The model under review builds one solid part; all positions refer to its coordinate system, in mm. Face numbers are marked on the shaded views. A direction names the side the tool comes from. Round coordinates to 2 decimals unless told otherwise and drop trailing zeros. Loops run counter-clockwise (first coordinate to the right, second up) from the corner with the lowest first, then second, coordinate; pieces in that order, holes last. Notation, with made-up numbers: M 1.25,73.5 L 57.25,73.5 A21 ccw 57.25,88.5 Z; hole C 25.5,-17.75 d3. An arc over 180 degrees is marked long. One line per question, with ' | ' between items.
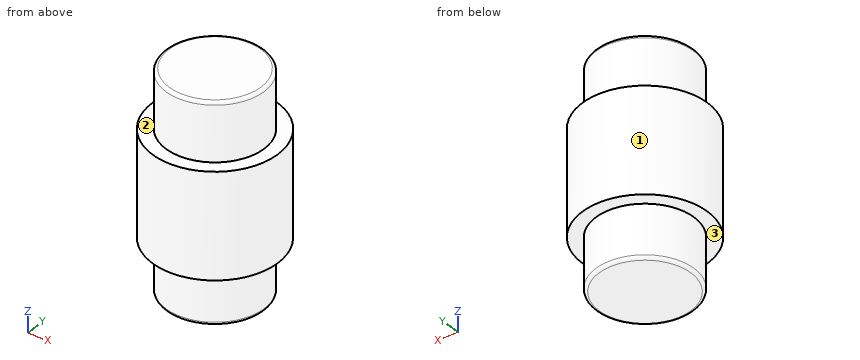
Autodesk Inventor part; units mm, degrees
ref_plane "YZ Plane" through (0, 0, 0) normal (1, 0, 0) x (0, 1, 0)
ref_plane "XZ Plane" through (0, 0, 0) normal (0, 1, 0) x (-1, 0, 0)
ref_plane "XY Plane" through (0, 0, 0) normal (0, 0, 1) x (1, 0, 0)
sketch "Sketch1" plane through (0, 0, 0) normal (0, 0, 1) x (1, 0, 0)
  circle A0 centre (0, 0) radius 4.7
  dimension "d0" = 9.4
extrude "Extrusion1" add sketch "Sketch1" along normal blind 5
sketch "Sketch2" plane through (0, 0, 5) normal (0, 0, 1) x (1, 0, 0)
  circle A0 centre (0, 0) radius 6
  dimension "d3" = 12
extrude "Extrusion2" add sketch "Sketch2" along normal blind 10
sketch "Sketch3" plane through (0, 0, 15) normal (0, 0, 1) x (1, 0, 0)
  circle A0 centre (0, 0) radius 4.7
  dimension "d6" = 9.4
extrude "Extrusion3" add sketch "Sketch3" along normal blind 5.556
fillet "Fillet1" radius 0.3 2 edges at (-4.7, 0, 20.556) (-4.7, 0, 0)
properties part number "eje escalonado V2"
1) Insertion check: P1, Ø5, axis at y = 4, z = 9, coming from the +X side; P2, Ø6, axis at y = 2.5, z = 3, coming from the -X side; P3, Ø2, axis at y = 0.5, z = 16.5, coming from the +X side. Each pin has a flat end and moves straight along its axis. Give the tip position at first contact, or say it passes through.
Output values:
P1: stops at x = 5.81 | P2: stops at x = -5.99 | P3: stops at x = 4.7
2) Machinability: for the marked faces 1, 2 and 3, which of the approach directions +Z, -Z, +X, -X, +Y, -Y give a long, thin tool a straight path to every point of the face, cutting with its end or side? Answer none if there is none.
Output values:
face 1: +Z, -Z | face 2: +Z | face 3: -Z
3) For line 1 (Y direction, x = 0, z = 18.25); line 2 (Z direction, x = 5, y = 1); line 3 (Y direction, x = 2.5, z = 5.75), list the stretches that pass through material, from the lowest coordinate up.
Output values:
line 1: y = -4.7 to 4.7 | line 2: z = 5 to 15 | line 3: y = -5.45 to 5.45
4) Add section C-C on z = 16.75. State the section outline as (x, y) points, then the cut area to 3 significant figures.
Output values:
outline: C 0,0 d9.4 | area: 69.4 mm²
5) Add section D-D on z = 11.25. State the section outline as (x, y) points, then the cut area to 3 significant figures.
Output values:
outline: C 0,0 d12 | area: 113 mm²
6) Add section A-A on x = 0. State the section outline as (y, z) points, then the cut area to 3 significant figures.
Output values:
outline: M -6,5 L -4.7,5 L -4.7,0.3 A0.3 ccw -4.4,0 L 4.4,0 A0.3 ccw 4.7,0.3 L 4.7,5 L 6,5 L 6,15 L 4.7,15 L 4.7,20.26 A0.3 ccw 4.4,20.56 L -4.4,20.56 A0.3 ccw -4.7,20.26 L -4.7,15 L -6,15 Z | area: 219 mm²
